For this review, take the finished solid that the model builds, in its own axes (mm). A direction names the side the tool comes from. Round coordinates to 2 decimals unless told otherwise and drop trailing zeros. Write each loop counter-clockwise with the first axis right and the second up, starting at its lowest first coordinate (ties: lowest second). Pieces come first, ordered by that corner, then holes. Notation, with made-up numbers: M -30.5,78.25 L 2.5,78.25 A26 cw 2.5,112.25 Z; hole C 81.25,74 d1. An arc over 180 degrees is marked long. Use one line per item in the form item = value. Start each with the question number.
Item 1: For faces 5 (the flat face through (-31.7, -9.7, 29.2)), 6 (the flat face through (-29.988, -4.938, 22.686)), 7 (the cylindrical face through (-42.33, -5.71, 86.91)), list the 3-axis set-ups (+Z, -Z, +X, -X, +Y, -Y) from which the entire face can be reached by the end or side of a thin tool; tool diameter is ignored.
Item 2: Draft analysis for pull direction Y (two halves, no side actions). For faces 1 (the flat face through (-31.47, -9.7, 67.05)), 2 (the cylindrical face through (-52.52, -4.39, 1.97)), 3 (the flat face through (-40, -5, 14)), 4 (the flat face through (-26, 0, 35)), state which applies: released by +Y, released by -Y, zero draft, split by the parting line, or undercut.
Item 3: Add section A-A (x = -54). State the section outline as (y, z) points, and give its area (3 significant figures).
Item 4: Add section D-D (z = 64.5). State the section outline as (x, y) points, and give its area (3 significant figures).
Item 5: Add section C-C (x = -24). State the section outline as (y, z) points, and give its area (3 significant figures).
Item 6: For P1, Ø4.5, axis at x = -53.5, y = -7, coming from the +Z side; P2, Ø6, axis at y = -5, z = 15.15, coming from the -X side; P3, Ø4.5, axis at y = -6, z = 62, coming from the +X side, all flat-tipped, find the tip position at first contact; note any pin that passes through.
Item 7: Add section B-B (z = 30.5). State the section outline as (x, y) points.
Item 8: For line 1 (Z direction, x = -41.2, y = -5); line 2 (X direction, y = -5, z = 2.05); line 3 (Y direction, x = -42.1, z = 15.15), list the stretches that pass through material, from the lowest coordinate up. Write a range as [from, to].
from build123d import *

# Parameters (mm, degrees)
PAD009_DEPTH    = 10
SKETCH021_R     = 2.35
POCKET008_DEPTH = 5
SKETCH022_R     = 1.6
POCKET009_DEPTH = 99.151
SKETCH023_R     = 3.25
POCKET010_DEPTH = 95.151
CHAMFER007_SIZE = 0.6
CHAMFER008_SIZE = 0.4


with BuildPart() as part:
    # Sketch020 → Pad009 (new body)
    with BuildSketch(Plane.XZ):
        Polygon((-60, 0), (0, 0), (0, 5), (-40, 99.15), (-45, 99.15), (-45, 5), (-60, 5), align=None)
        Polygon((-40, 5), (-5.4325428768, 5), (-20.2529345059, 39.8834967971), align=None, mode=Mode.SUBTRACT)
        Polygon((-40, 15.1496021181), (-22.7162714384, 45.6815761019), (-40, 86.3631522038), align=None, mode=Mode.SUBTRACT)
    extrude(amount=PAD009_DEPTH)

    # Sketch021 (on Face5 of Pad009) → Pocket008 (cut)
    with BuildSketch(Plane(origin=(-45, 0, 0), x_dir=(0, 0, -1), z_dir=(-1, 0, 0))):
        with Locations((-89.15, 5)):
            Circle(SKETCH021_R)
        with Locations((-15.15, 5)):
            Circle(SKETCH021_R)
    extrude(amount=-POCKET008_DEPTH, mode=Mode.SUBTRACT)

    # Sketch022 (on Face1 of Pocket008) → Pocket009 (cut, through all)
    with BuildSketch(Plane(origin=(0, 0, 0), x_dir=(1, 0, 0), z_dir=(0, 0, -1))):
        with Locations((-54, 5)):
            Circle(SKETCH022_R)
        with Locations((-6, 5)):
            Circle(SKETCH022_R)
    extrude(amount=-POCKET009_DEPTH, mode=Mode.SUBTRACT)

    # Sketch023 (on Sketch) → Pocket010 (cut, through all)
    with BuildSketch(Plane(origin=(0, 0, 4), x_dir=(1, 0, 0), z_dir=(0, 0, -1))):
        with Locations((-54, 5)):
            Circle(SKETCH023_R)
        with Locations((-6, 5)):
            Circle(SKETCH023_R)
    extrude(amount=-POCKET010_DEPTH, mode=Mode.SUBTRACT)

    # Chamfer007
    chamfer007_edges = [part.edges().sort_by_distance(p)[0] for p in [
        (-30, 0, 0),
        (0, 0, 2.5),
        (-20, 0, 52.075),
        (-42.5, 0, 99.15),
        (-45, 0, 52.075),
        (-52.5, 0, 5),
        (-60, 0, 2.5),
        (-31.358136, 0, 30.415589),
        (-31.358136, 0, 66.022364),
        (-40, 0, 50.756377),
        (-22.716271, 0, 5),
        (-12.842739, 0, 22.441748),
        (-30.126467, 0, 22.441748),
        (-30, -10, 0),
        (0, -10, 2.5),
        (-20, -10, 52.075),
        (-42.5, -10, 99.15),
        (-45, -10, 52.075),
        (-52.5, -10, 5),
        (-60, -10, 2.5),
        (-31.358136, -10, 30.415589),
        (-31.358136, -10, 66.022364),
        (-40, -10, 50.756377),
        (-22.716271, -10, 5),
        (-12.842739, -10, 22.441748),
        (-30.126467, -10, 22.441748),
        (-40, -5, 99.15),
        (-45, -5, 99.15),
        (-60, -5, 5),
        (-60, -5, 0),
        (0, -5, 0),
        (0, -5, 5),
    ]]
    chamfer(chamfer007_edges, length=CHAMFER007_SIZE)

    # Chamfer008
    chamfer008_edges = [part.edges().sort_by_distance(p)[0] for p in [
        (-45, -5, 91.5),
        (-45, -5, 17.5),
    ]]
    chamfer(chamfer008_edges, length=CHAMFER008_SIZE)


solid = part.part
Calculated:
q1.face_5 = -Y
q1.face_6 = +Y, -Y
q1.face_7 = -X
q2.face_1 = released by -Y
q2.face_2 = undercut
q2.face_3 = undercut
q2.face_4 = released by +Y
q3.outline = M -10,0.6 L -9.4,0 L -6.6,0 L -6.6,4 L -8.25,4 L -8.25,5 L -9.4,5 L -10,4.4 Z; M -3.4,0 L -0.6,0 L 0,0.6 L 0,4.4 L -0.6,5 L -1.75,5 L -1.75,4 L -3.4,4 Z
q3.area = 30.0 mm^2
q4.outline = M -45,-9.4 L -44.4,-10 L -40.6,-10 L -40,-9.4 L -40,-0.6 L -40.6,0 L -44.4,0 L -45,-0.6 Z; M -30.71,-9.4 L -30.06,-10 L -25.93,-10 L -25.28,-9.4 L -25.28,-0.6 L -25.93,0 L -30.06,0 L -30.71,-0.6 Z
q4.area = 103 mm^2
q5.outline = M -10,0.6 L -9.4,0 L -0.6,0 L 0,0.6 L 0,4.4 L -0.6,5 L -9.4,5 L -10,4.4 Z; M -10,34.48 L -9.4,33.26 L -0.6,33.26 L 0,34.48 L 0,42.2 L -0.6,43.41 L -9.4,43.41 L -10,42.2 Z; M -10,50.24 L -9.4,48.7 L -0.6,48.7 L 0,50.24 L 0,59.96 L -0.6,61.49 L -9.4,61.49 L -10,59.96 Z
q5.area = 275 mm^2
q6.P1 = 5
q6.P2 = -45
q6.P3 = -23.26
q7.outline = M -45,-9.4 L -44.4,-10 L -40.6,-10 L -40,-9.4 L -40,-0.6 L -40.6,0 L -44.4,0 L -45,-0.6 Z; M -31.31,-9.4 L -30.62,-10 L -26.25,-10 L -25.56,-9.4 L -25.56,-0.6 L -26.25,0 L -30.62,0 L -31.31,-0.6 Z; M -16.27,-9.4 L -15.61,-10 L -11.49,-10 L -10.83,-9.4 L -10.83,-0.6 L -11.49,0 L -15.61,0 L -16.27,-0.6 Z
q8.line_1 = [0, 12.8], [17.5, 86.8], [91.5, 99.15]
q8.line_2 = [-60, -55.6], [-52.4, -7.6], [-4.4, 0]
q8.line_3 = [-10, -7.35], [-2.65, 0]
